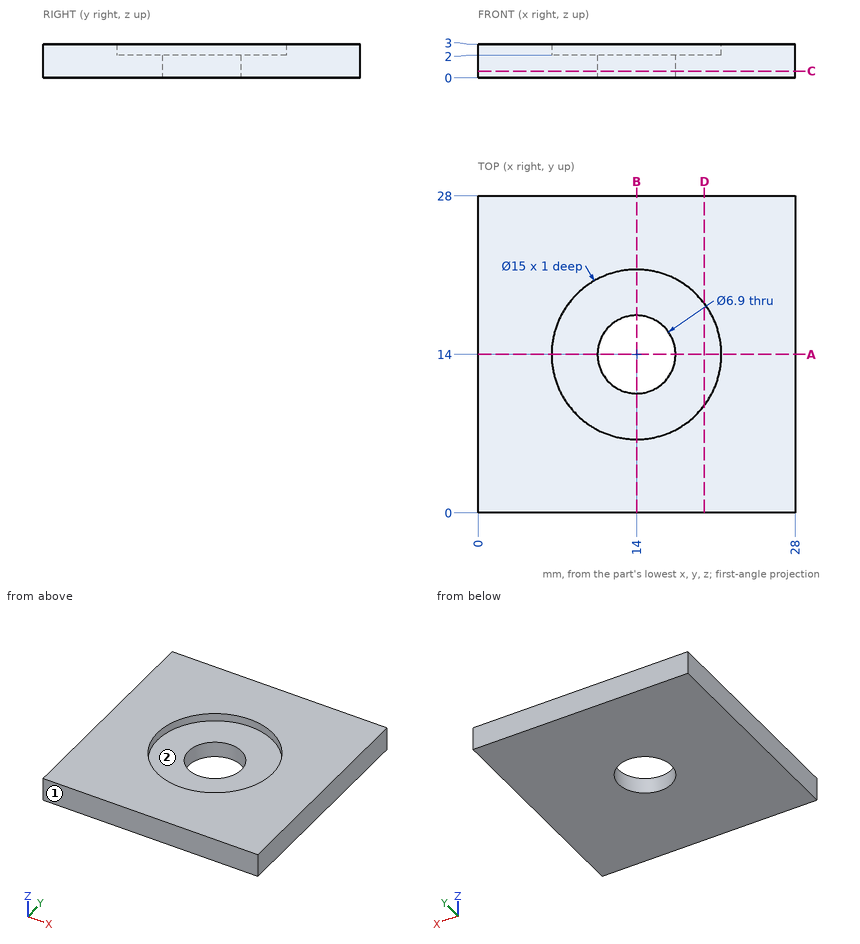
Study the drawing (mm; zero at the part's minimum x, y, z) and answer. Round coordinates to 2 decimals unless told otherwise and drop trailing zeros. Loops run counter-clockwise (first coordinate to the right, second up) from the corner with the lowest first, then second, coordinate; pieces in that order, holes last. Notation, with made-up numbers: (-23.75, -22) - (25.25, -22) arc R21 cw to (25.25, 17) - close; hole circle Ø9 at (-23, 26). An arc over 180 degrees is marked (long way). Use one line per item in the form item = value. Start each with the question number.
1. The part is cut by section C-C on z = 0.6. Determine the outline of the cut face in (x, y).
2. The part is cut by section D-D on x = 20. Determine the outline of the cut face in (y, z), then the cut area to 3 significant figures.
3. The part is cut by section A-A on y = 14. Determine the outline of the cut face in (x, z).
4. Consider line 1 (Y direction, x = 14, z = 2.75); line 2 (Y direction, x = 14, z = 0.95); line 3 (X direction, y = 11.25, z = 1.6). Determine where each line is inside the solid, lowest interval first. Write a range as [from, to].
5. For a pull along X with two mould halves and no side action, classify the marked faces 1 and 2 as pulls with the +X half, pulls with the -X half, needs draft (parallel to the pull), parting line crosses it, or undercut.
6. Given pin 1 Ø11 at (x, y) = (14, 14) entering from -Z; pin 2 Ø3 at (x, y) = (12, 11) entering from +Z, each flat-ended and moving along its own axis, determine where each tip first touches the part or whether it passes through.
Geometry check:
q1.outline = (0, 0) - (28, 0) - (28, 28) - (0, 28) - close; hole circle Ø6.9 at (14, 14)
q2.outline = (0, 0) - (28, 0) - (28, 3) - (18.5, 3) - (18.5, 2) - (9.5, 2) - (9.5, 3) - (0, 3) - close
q2.area = 75.0 mm^2
q3.outline = (0, 0) - (10.55, 0) - (10.55, 2) - (6.5, 2) - (6.5, 3) - (0, 3) - close; (17.45, 0) - (28, 0) - (28, 3) - (21.5, 3) - (21.5, 2) - (17.45, 2) - close
q4.line_1 = [0, 6.5], [21.5, 28]
q4.line_2 = [0, 10.55], [17.45, 28]
q4.line_3 = [0, 11.92], [16.08, 28]
q5.face_1 = needs draft
q5.face_2 = undercut
q6.pin_1 = 0
q6.pin_2 = 2
